Could you check a few things on this drawing? It's one solid part, dimensions in mm from its lowest x, y, z. A direction names the side the tool comes from. Give positions to 0.01 mm unless a question says otherwise; leave off trailing zeros. Order: outer loops, then holes, each group sorted by start corner. A loop starts at its lowest first (then second) coordinate and runs counter-clockwise, first axis right, second up.
(1) Imagine slicing it at D-D, the plane x = 5.5. Write out the boundary of the cut face in (y, z), then the cut area to 3 significant figures.
(2) Imagine slicing it at A-A, the plane y = 5.75. Write out the boundary of the cut face in (x, z), then the cut area to 3 significant figures.
(3) If we mould it in two halves opening along Y, with no side actions, what happens to the marked faces 4, 5, 6 and 7? For each: released by +Y, released by -Y, zero draft, split by the parting line, or undercut.
(4) Will these pins go through, and if not, where does the flat tip stop? pin 1 (0.9 mm diameter, centred on y = 1, z = 10, fed in from -X); pin 2 (4 mm diameter, centred on x = 8, z = 15, fed in from -Y); pin 3 (2.5 mm diameter, centred on x = 11, z = 8.5, fed in from +Y); pin 4 (2 mm diameter, centred on x = 19.5, z = 5, fed in from +Y).
(5) Imagine slicing it at B-B, the plane x = 17.25. Write out the boundary of the cut face in (y, z), then the cut area to 3 significant figures.
(6) Imagine slicing it at C-C, the plane y = 13. Write out the boundary of the cut face in (x, z), then the cut area to 3 significant figures.
(7) On a 3-axis mill with a long thin cutter (end or side, diameter ignored), from which of +Z, -Z, +X, -X, +Y, -Y can I reach the whole of each face in a straight line? I mean the marked faces 1, 2 and 3. Say none if no direction works.
(8) If I drill on probe 1 along X at (y, z) = (7, 10); probe 2 along Y at (x, z) = (6, 17.25); probe 3 along X at (y, z) = (5.5, 2), over which ranges is the centre line in solid material (lowest first)?
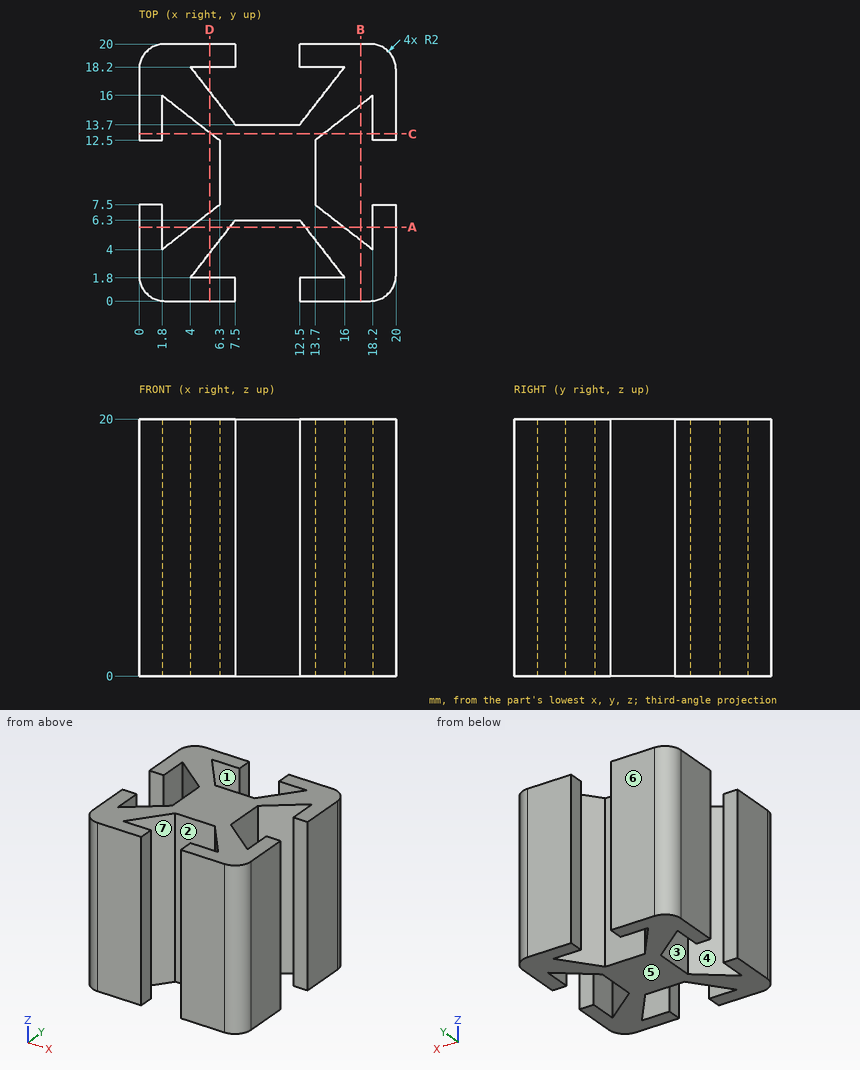
Answer block:
1. outline: (0, 0) - (1.8, 0) - (1.8, 20) - (0, 20) - close; (3.73, 0) - (6.88, 0) - (6.88, 20) - (3.73, 20) - close; (13.12, 0) - (16.27, 0) - (16.27, 20) - (13.12, 20) - close; (18.2, 0) - (20, 0) - (20, 20) - (18.2, 20) - close
1. area: 198 mm2
2. outline: (0, 0) - (1.8, 0) - (1.8, 20) - (0, 20) - close; (4.05, 0) - (7.07, 0) - (7.07, 20) - (4.05, 20) - close; (12.93, 0) - (15.95, 0) - (15.95, 20) - (12.93, 20) - close; (18.2, 0) - (20, 0) - (20, 20) - (18.2, 20) - close
2. area: 193 mm2
3. face 4: undercut
3. face 5: zero draft
3. face 6: released by +Y
3. face 7: undercut
4. pin 1: stops at x = 0.08
4. pin 2: stops at y = 0
4. pin 3: stops at y = 13.7
4. pin 4: stops at y = 19.94
5. outline: (0, 0) - (4.74, 0) - (4.74, 20) - (0, 20) - close; (15.26, 0) - (20, 0) - (20, 20) - (15.26, 20) - close
5. area: 190 mm2
6. outline: (0, 0) - (1.8, 0) - (1.8, 20) - (0, 20) - close; (5.66, 0) - (14.34, 0) - (14.34, 20) - (5.66, 20) - close; (18.2, 0) - (20, 0) - (20, 20) - (18.2, 20) - close
6. area: 246 mm2
7. face 1: +Z, -Z
7. face 2: +Z, -Z, -Y
7. face 3: +Z, -Z, -X
8. probe 1: x = 0 to 1.8, 5.66 to 14.34, 18.2 to 20
8. probe 2: y = 0 to 1.8, 4.37 to 7.27, 12.73 to 15.63, 18.2 to 20
8. probe 3: x = 0 to 1.8, 3.73 to 6.88, 13.12 to 16.27, 18.2 to 20
